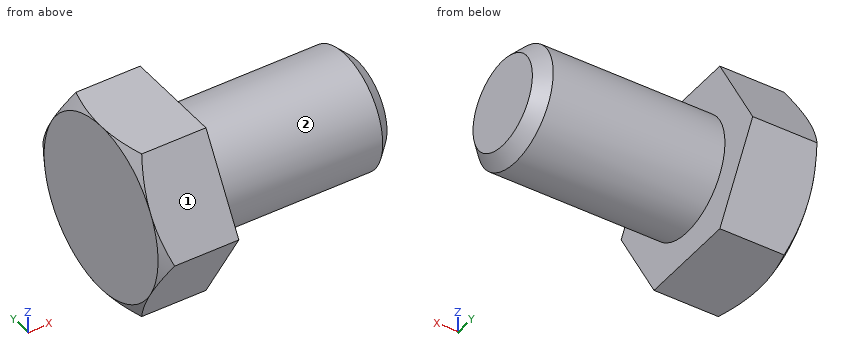
from build123d import *

# Parameters (mm, degrees)
SKETCH5_R           = 7.9375
BOSS_EXTRUDE3_DEPTH = 25.4
CHAMFER1_SIZE       = 1.731818182
BOSS_EXTRUDE4_DEPTH = 9.921875
SKETCH8_OUTSIDE_W   = 161.776
SKETCH8_OUTSIDE_H   = 165.46
SKETCH8_OUTSIDE_R   = 11.90625
CUT_EXTRUDE3_DEPTH  = 36.321875
CUT_EXTRUDE3_TAPER  = 60


with BuildPart() as part:
    # Sketch5 → Boss-Extrude3 (new body)
    with BuildSketch(Plane(origin=(17.6609375, 0, 0), x_dir=(0, 0, -1), z_dir=(1, 0, 0))):
        Circle(SKETCH5_R)
    extrude(amount=-BOSS_EXTRUDE3_DEPTH)

    # Chamfer1
    chamfer1_edges = [part.edges().sort_by_distance(p)[0] for p in [
        (17.6609375, 0, 7.9375),
    ]]
    chamfer(chamfer1_edges, length=CHAMFER1_SIZE)

    # Sketch6 → Boss-Extrude4 (add)
    with BuildSketch(Plane.ZY.offset(7.7390625)):
        Polygon((11.90625, 6.874076643), (0, 13.748153285), (-11.90625, 6.874076643), (-11.90625, -6.874076643), (0, -13.748153285), (11.90625, -6.874076643), align=None)
    extrude(amount=BOSS_EXTRUDE4_DEPTH)

    # Sketch8 outside → Cut-Extrude3 (cut, through all)
    with BuildSketch(Plane.ZY.offset(17.6609375)):
        Rectangle(SKETCH8_OUTSIDE_W, SKETCH8_OUTSIDE_H)
        Circle(SKETCH8_OUTSIDE_R, mode=Mode.SUBTRACT)
    extrude(amount=-CUT_EXTRUDE3_DEPTH, taper=CUT_EXTRUDE3_TAPER, mode=Mode.SUBTRACT)


solid = part.part
The model under review builds one solid part; all positions refer to its coordinate system, in mm. Face numbers are marked on the shaded views. A direction names the side the tool comes from. Round coordinates to 2 decimals unless told otherwise and drop trailing zeros. Write each loop counter-clockwise with the first axis right and the second up, starting at its lowest first coordinate (ties: lowest second). Pieces come first, ordered by that corner, then holes. Notation, with made-up numbers: (31, -13) - (48, -13) arc R8 cw to (48, 1) - close; hole circle Ø3 at (-29.5, 85.5). An arc over 180 degrees is marked (long way). One line per item, written item: value. Start each with the question number.
1. Machinability: for the marked faces 1 and 2, which of the approach directions +Z, -Z, +X, -X, +Y, -Y give a long, thin tool a straight path to every point of the face, cutting with its end or side? Answer none if there is none.
2. To check wall thickness, follow L1, parallel to X at y = 7.75, z = -8.25; L2, parallel to X at y = 4.75, z = 4; L3, parallel to Y at x = -4.5, z = 0.25. State the ranges of each line that lie inside material, in increasing order. Write a range as from..to.
3. Clearance check with flat-ended pins moving along their axes: P1, Ø12, axis at x = 4.5, z = 7, coming from the -Y side; P2, Ø1, axis at x = 9, z = -2.5, coming from the -Y side; P3, Ø10, axis at x = -9.5, y = -10, coming from the -Z side. State where each tip first meets the part, or that it passes through.
4. Consider section A-A on x = -14. Write out the cut boundary in (y, z).
5. Consider section B-B on x = -5.5. Write out the cut boundary in (y, z) (1 decimal).
Checks:
1. face 1: +Z, +X, -X, -Y
1. face 2: +X
2. L1: x = -17.66..-7.74
2. L2: x = -17.66..17.66
2. L3: y = -7.93..7.93
3. P1: stops at y = -7.87
3. P2: stops at y = -7.68
3. P3: stops at z = -11.91
4. outline: (-13.75, 0) - (-6.87, -11.91) - (6.87, -11.91) - (13.75, 0) - (6.87, 11.91) - (-6.87, 11.91) - close
5. outline: circle Ø15.9 at (0, 0)
